```python
from build123d import *

# Parameters (mm, degrees)
F0_W     = 1018
F0_H     = 500
F1_DEPTH = 19.2
F3_DEPTH = 3
F4_DEPTH = 19.2


with BuildPart() as f1:
    # F0 (on Top) → F1 (new body)
    with BuildSketch(Plane.XY):
        with Locations((9, 0)):
            Rectangle(F0_W, F0_H)
    extrude(amount=F1_DEPTH)

    # F2 (on face) → F3 (cut)
    with BuildSketch(Plane.XY.offset(19.2)):
        with BuildLine():
            ThreePointArc((150, 118.65), (148.140128, 123.140128), (143.65, 125))
            Line((143.65, 125), (-143.65, 125))
            ThreePointArc((-143.65, 125), (-148.140128, 123.140128), (-150, 118.65))
            Line((-150, 118.65), (-150, -118.65))
            ThreePointArc((-150, -118.65), (-148.140128, -123.140128), (-143.65, -125))
            Line((-143.65, -125), (143.65, -125))
            ThreePointArc((143.65, -125), (148.140128, -123.140128), (150, -118.65))
            Line((150, -118.65), (150, 118.65))
        make_face()
        with BuildLine():
            Line((-135, -103.65), (-135, 103.65))
            ThreePointArc((-135, 103.65), (-133.140128, 108.140128), (-128.65, 110))
            Line((-128.65, 110), (128.65, 110))
            ThreePointArc((128.65, 110), (133.140128, 108.140128), (135, 103.65))
            Line((135, 103.65), (135, -103.65))
            ThreePointArc((135, -103.65), (133.140128, -108.140128), (128.65, -110))
            Line((128.65, -110), (-128.65, -110))
            ThreePointArc((-128.65, -110), (-133.140128, -108.140128), (-135, -103.65))
        make_face(mode=Mode.SUBTRACT)
    extrude(amount=-F3_DEPTH, mode=Mode.SUBTRACT)

    # F2 (on face) → F4 (cut, through all)
    with BuildSketch(Plane.XY.offset(19.2)):
        with BuildLine():
            ThreePointArc((-128.65, 110), (-133.140128, 108.140128), (-135, 103.65))
            Line((-135, 103.65), (-135, -103.65))
            ThreePointArc((-135, -103.65), (-133.140128, -108.140128), (-128.65, -110))
            Line((-128.65, -110), (128.65, -110))
            ThreePointArc((128.65, -110), (133.140128, -108.140128), (135, -103.65))
            Line((135, -103.65), (135, 103.65))
            ThreePointArc((135, 103.65), (133.140128, 108.140128), (128.65, 110))
            Line((128.65, 110), (-128.65, 110))
        make_face()
    extrude(amount=-F4_DEPTH, mode=Mode.SUBTRACT)


solid = f1.part
```
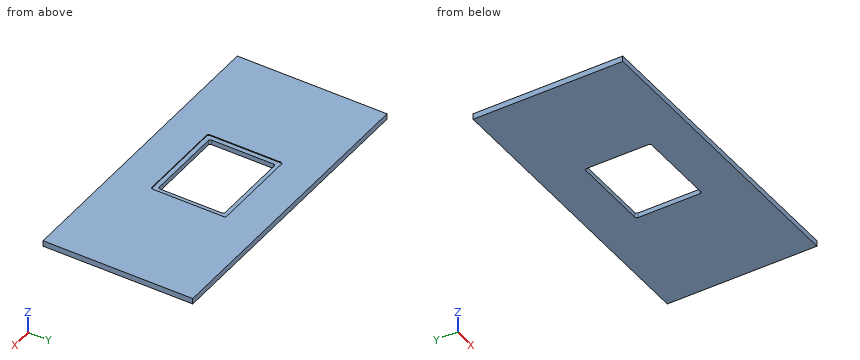
Part model, mm, in its own coordinate system. Round coordinates to 2 decimals unless told otherwise and drop trailing zeros. Write each loop counter-clockwise with the first axis right and the second up, starting at its lowest first coordinate (ties: lowest second). Pieces come first, ordered by that corner, then holes. Notation, with made-up numbers: (-21, 53.5) -> (17, 53.5) arc R28 cw to (17, 88.5) -> close; hole circle Ø6 at (-25, -8.75). An arc over 180 degrees is marked (long way). Return JSON: item names as keys, results as strings. Group by question number.
Q1. Saw through at A-A on y = -57. Write the cut outline in (x, z), plus the area to 3 significant figures.
Q2. Saw through at B-B on x = -65.5. Write the cut outline in (y, z).
Q3. Probe L1, parallel to X at y = -19.5, z = 9.5; L2, parallel to Y at x = 94, z = 8; L3, parallel to Y at x = 133, z = 9.25. List the from-to ranges inside material, lowest first. Write a range as [from, to].
Q4. Saw through at C-C on z = 9.75. Write the cut outline in (x, y).
Answer:
{
 "1": {"outline": "(-500, 0) -> (-135, 0) -> (-135, 16.2) -> (-150, 16.2) -> (-150, 19.2) -> (-500, 19.2) -> close; (135, 0) -> (518, 0) -> (518, 19.2) -> (150, 19.2) -> (150, 16.2) -> (135, 16.2) -> close", "area": "14,300 mm2"},
 "2": {"outline": "(-250, 0) -> (-110, 0) -> (-110, 16.2) -> (-125, 16.2) -> (-125, 19.2) -> (-250, 19.2) -> close; (110, 0) -> (250, 0) -> (250, 19.2) -> (125, 19.2) -> (125, 16.2) -> (110, 16.2) -> close"},
 "3": {"L1": "[-500, -135], [135, 518]", "L2": "[-250, -110], [110, 250]", "L3": "[-250, -108.28], [108.28, 250]"},
 "4": {"outline": "(-500, -250) -> (518, -250) -> (518, 250) -> (-500, 250) -> close; hole (-135, -103.65) arc R6.35 ccw to (-128.65, -110) -> (128.65, -110) arc R6.35 ccw to (135, -103.65) -> (135, 103.65) arc R6.35 ccw to (128.65, 110) -> (-128.65, 110) arc R6.35 ccw to (-135, 103.65) -> close"}
}
